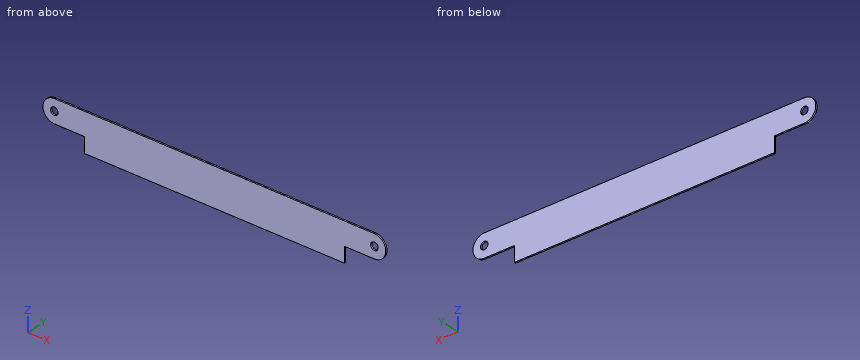
from build123d import *

# Parameters (mm, degrees)
SKETCH1_R           = 2.5
BOSS_EXTRUDE1_DEPTH = 1


with BuildPart() as part:
    # Sketch1 → Boss-Extrude1 (new body)
    with BuildSketch(Plane(origin=(0, 0, 0), x_dir=(1, 0, 0), z_dir=(0, 1, 0))):
        with BuildLine():
            Line((0, 7.5), (20, 7.5))
            Line((20, 7.5), (20, 17.5))
            Line((20, 17.5), (192.13, 17.5))
            Line((192.13, 17.5), (192.13, 7.5))
            Line((192.13, 7.5), (212.13, 7.5))
            ThreePointArc((212.13, 7.5), (219.63, 0), (212.13, -7.5))
            Line((212.13, -7.5), (0, -7.5))
            ThreePointArc((0, -7.5), (-7.5, 0), (0, 7.5))
        make_face()
        with Locations(Location((0, 0, 0), (0, 0, 270))):
            Circle(SKETCH1_R, mode=Mode.SUBTRACT)
        with Locations(Location((212.13, 0, 0), (0, 0, 270))):
            Circle(SKETCH1_R, mode=Mode.SUBTRACT)
    extrude(amount=BOSS_EXTRUDE1_DEPTH)


solid = part.part
Source: CAD feature listing. Evaluate the final solid. Frame: model axes, mm. Round coordinates to 2 decimals unless told otherwise and drop trailing zeros. Write each loop counter-clockwise with the first axis right and the second up, starting at its lowest first coordinate (ties: lowest second). Pieces come first, ordered by that corner, then holes. Notation, with made-up numbers: M 22,47 L 29,47 A33 ccw 29,86 Z; hole C 86.25,2.25 d10. An arc over 180 degrees is marked long. One line per item, written item: value. Start each with the question number.
Item 1: Section query D-D (x = 9). Return the cut outline in (y, z), plus the area to 3 significant figures.
Item 2: Pin query (flat end, axial travel): pin 1 (0.5 mm diameter, centred on x = 8, y = 0.5, fed in from -Z). Return the tip coordinate at first contact, or that it passes through.
Item 3: Section query C-C (z = -10). Return the cut outline in (x, y), plus the area to 3 significant figures.
Item 4: Section query B-B (z = 0). Return the cut outline in (x, y).
Item 5: Ray query, L1, parallel to X at y = 0.6, z = 0; L2, parallel to Z at x = 212.13, y = 0.5; L3, parallel to Z at x = 204.5, y = 0.55. Return the intervals inside material, ascending. Write a range as from..to.
Item 6: Section query A-A (y = 0.4). Return the cut outline in (x, z).
Result set:
1. outline: M 0,-7.5 L 1,-7.5 L 1,7.5 L 0,7.5 Z
1. area: 15.0 mm²
2. pin 1: stops at z = -7.5
3. outline: M 20,0 L 192.13,0 L 192.13,1 L 20,1 Z
3. area: 172 mm²
4. outline: M -7.5,0 L -2.5,0 L -2.5,1 L -7.5,1 Z; M 2.5,0 L 209.63,0 L 209.63,1 L 2.5,1 Z; M 214.63,0 L 219.63,0 L 219.63,1 L 214.63,1 Z
5. L1: x = -7.5..-2.5, 2.5..209.63, 214.63..219.63
5. L2: z = -7.5..-2.5, 2.5..7.5
5. L3: z = -7.5..7.5
6. outline: M 0,-7.5 L 20,-7.5 L 20,-17.5 L 192.13,-17.5 L 192.13,-7.5 L 212.13,-7.5 A7.5 ccw 212.13,7.5 L 0,7.5 A7.5 ccw Z; hole C 0,0 d5; hole C 212.13,0 d5
